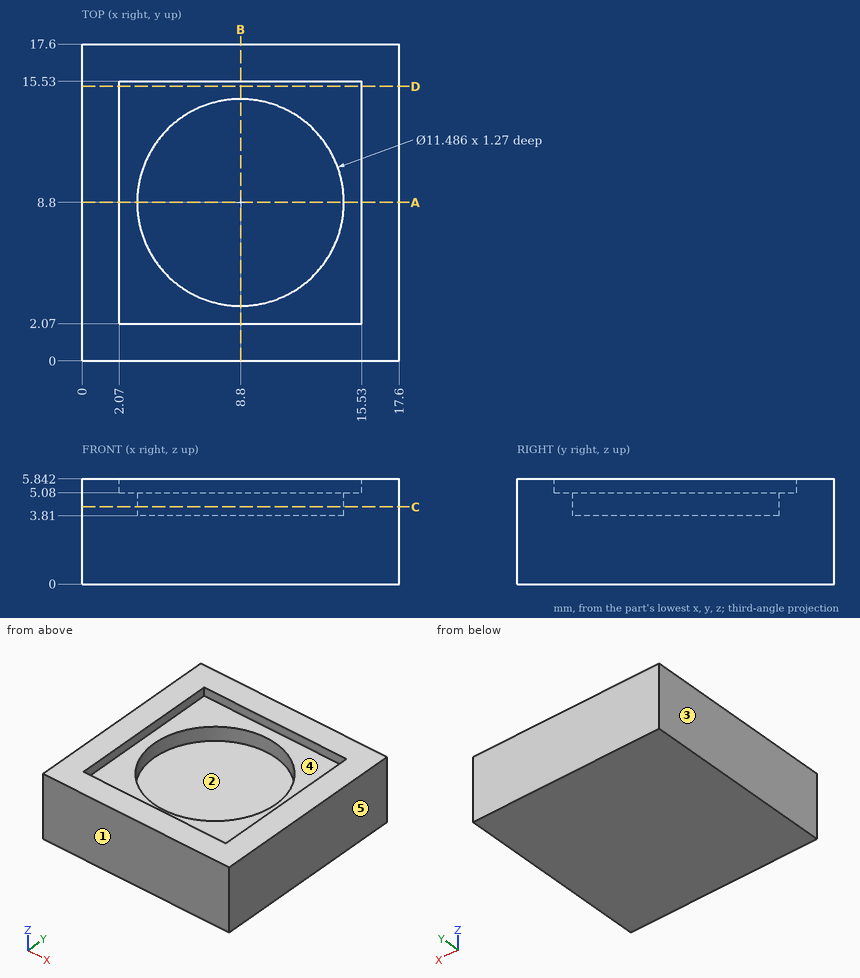
Input: dimensioned drawing with shaded views. Units: mm. Origin: part minimum x, y, z. A direction names the side the tool comes from. Coordinates: 2 decimals unless noted, no trailing zeros. Loops run counter-clockwise (first coordinate to the right, second up) from the corner with the lowest first, then second, coordinate; pieces in that order, holes last. Notation, with made-up numbers: M -12,74.5 L -7,74.5 A19 ccw -7,81.5 Z; hole C 68,89 d1. An arc over 180 degrees is marked long. One line per item, written item: value. Start each with the question number.
1) Reachability of the marked faces 4 and 5 from +Z, -Z, +X, -X, +Y, -Y: full face, straight path, thin tool, end or side. Return the list, or none.
2) Cut plane C-C (z = 4.3). Return loops of the section in (x, y), then the cut area to 3 significant figures.
3) Pin query (flat end, axial travel): P1, Ø1, axis at x = 13, y = 12.5, coming from the +Z side; P2, Ø6, axis at x = 5, y = 7, coming from the -Z side; P3, Ø5, axis at x = 9.5, y = 9.5, coming from the +Z side. Return the tip coordinate at first contact, or that it passes through.
4) Cut plane D-D (y = 15.25). Return loops of the section in (x, z).
5) Material intervals for L1, parallel to X at y = 13.5, z = 5.45; L2, parallel to Y at x = 8.8, z = 4.8; L3, parallel to Z at x = 11.5, y = 5, sorted ascending. Write a range as from..to.
6) Cut plane A-A (y = 8.8). Return loops of the section in (x, z).
7) Draft query along X for the marked faces 1, 2 and 3. Return one class per face: released by +X, released by -X, zero draft, split by the parting line, or undercut.
Evaluation:
1. face 4: +Z
1. face 5: +Z, -Z, +X, +Y, -Y
2. outline: M 0,0 L 17.6,0 L 17.6,17.6 L 0,17.6 Z; hole C 8.8,8.8 d11.49
2. area: 206 mm^2
3. P1: z = 5.08
3. P2: z = 0
3. P3: z = 3.81
4. outline: M 0,0 L 17.6,0 L 17.6,5.84 L 15.53,5.84 L 15.53,5.08 L 2.07,5.08 L 2.07,5.84 L 0,5.84 Z
5. L1: 0..2.07, 15.53..17.6
5. L2: 0..3.06, 14.54..17.6
5. L3: 0..3.81
6. outline: M 0,0 L 17.6,0 L 17.6,5.84 L 15.53,5.84 L 15.53,5.08 L 14.54,5.08 L 14.54,3.81 L 3.06,3.81 L 3.06,5.08 L 2.07,5.08 L 2.07,5.84 L 0,5.84 Z
7. face 1: zero draft
7. face 2: undercut
7. face 3: released by -X
